Autodesk Inventor part; units mm, degrees
ref_plane "YZ Plane" through (0, 0, 0) normal (1, 0, 0) x (0, 1, 0)
ref_plane "XZ Plane" through (0, 0, 0) normal (0, 1, 0) x (-1, 0, 0)
ref_plane "XY Plane" through (0, 0, 0) normal (0, 0, 1) x (1, 0, 0)
sketch "草图1" plane through (0, 0, 0) normal (0, 0, 1) x (1, 0, 0)
  circle A0 centre (0, 0) radius 15
  circle A1 centre (0, 150) radius 5
  line L0 (0, 150) -> (0, 0)
  line L1 (-14.96663, 1) -> (-4.988877, 150.333333)
  line L2 (4.988877, 150.333333) -> (14.96663, 1)
  dimension "d0" = 30
  dimension "d1" = 10
  dimension "d2" = 150
extrude "拉伸1" add sketch "草图1" along normal blind 15
sketch "草图2" plane through (0, 0, 15) normal (0, 0, 1) x (1, 0, 0)
  circle A0 centre (0, 0) radius 7.5
  dimension "d5" = 15
extrude "拉伸2" cut sketch "草图2" against normal through all
sketch "草图3" plane through (0, 0, 15) normal (0, 0, 1) x (1, 0, 0)
  circle A0 centre (0, 150) radius 5
  arc A1 (4.988877, 150.333333) -> (-4.988877, 150.333333) centre (0, 150) ccw
  point P0 (0, 0)
  dimension "d8" = 10
extrude "拉伸3" add sketch "草图3" along normal blind 42.5
thread "螺纹1"
chamfer "倒角1" distance 0.25 angle 45 1 edges at (-5, 150, 57.5)
chamfer "倒角2" distance 1 angle 45 7 edges at (9.9778, 75.6667, 15) (0, -15, 15) (-9.9778, 75.6667, 15) (9.9778, 75.6667, 0) (0, 155, 0) (-9.9778, 75.6667, 0) (0, -15, 0)
chamfer "倒角3" distance 0.25 angle 45 1 edges at (-5, 150, 57.25)
equation "\"d6\" = d5"
properties part number "刀轴带动盘连杆"
Source: CAD feature listing. Evaluate the final solid. Frame: model axes, mm. A direction names the side the tool comes from. Coordinates: 2 decimals unless noted, no trailing zeros. Write each loop counter-clockwise with the first axis right and the second up, starting at its lowest first coordinate (ties: lowest second). Pieces come first, ordered by that corner, then holes. Notation, with made-up numbers: (-35, 85) -> (-6, 85) arc R30 cw to (-6, 115) -> close; hole circle Ø4 at (-27, 52). An arc over 180 degrees is marked (long way). Return JSON: item names as keys, results as strings. Group by question number.
1) Section query B-B, the plane y = 31. Return loops of the section in (x, z), plus the area to 3 significant figures.
2) Contact query for flat-ended pins moving along their axis: P1, Ø1.5, axis at y = 29.5, z = 10.5, coming from the -X side; P2, Ø1, axis at x = -6.5, y = 131, coming from the -Z side; P3, Ø8, axis at x = -11.5, y = 3, coming from the +Z side. Output: stop coordinate, or through.
3) Section query C-C, the plane z = 30. Return loops of the section in (x, y), plus the area to 3 significant figures.
4) Section query A-A, the plane z = 7.5. Return loops of the section in (x, y), plus the area to 3 significant figures.
5) Set-up query: faces 1 (the face through (0, 150, 57.5)), 2 (the face through (2.26, 154.46, 28.61)). Return all of +Z, -Z, +X, -X, +Y, -Y with unobstructed straight access to the full face (end or side cutting, diameter ignored); none if empty.
6) Mould query, pull axis X, two halves, no side actions, for faces 3 (the face through (-7.493, 0.33, 7.605)), 4 (the face through (0.325, -14.17, 14.826)), 5 (the face through (9.91, 76.71, 7.41)), 6 (the face through (0, 50, 15)). Classes: +X half, -X half, draft (parallel to the pull), parting line (faces both ways), or undercut.
7) Section query D-D, the plane y = 54.5. Return loops of the section in (x, z).
8) Ray query, line 1 along Y through (x, z) = (0, 3); line 2 along Z through (x, y) = (-5.25, 6); line 3 along Y through (x, z) = (-0.25, 47). Return the intervals inside material, ascending.
From the geometry:
{
 "1": {"outline": "(-12.96, 1) -> (-11.96, 0) -> (11.96, 0) -> (12.96, 1) -> (12.96, 14) -> (11.96, 15) -> (-11.96, 15) -> (-12.96, 14) -> close", "area": "387 mm²"},
 "2": {"P1": "x = -13.11", "P2": "z = 0.72", "P3": "z = 15"},
 "3": {"outline": "circle Ø10 at (0, 150)", "area": "78.5 mm²"},
 "4": {"outline": "(-14.97, 1) arc R15 ccw (long way) to (14.97, 1) -> (4.99, 150.33) arc R5 ccw to (-4.99, 150.33) -> close; hole circle Ø15 at (0, 0)", "area": "3,220 mm²"},
 "5": {"face 1": "+Z, +X, -X, +Y, -Y", "face 2": "+Z"},
 "6": {"face 3": "undercut", "face 4": "parting line", "face 5": "+X half", "face 6": "draft"},
 "7": {"outline": "(-11.39, 1) -> (-10.39, 0) -> (10.39, 0) -> (11.39, 1) -> (11.39, 14) -> (10.39, 15) -> (-10.39, 15) -> (-11.39, 14) -> close"},
 "8": {"line 1": "-15 to -7.5, 7.5 to 155", "line 2": "0 to 15", "line 3": "145.01 to 154.99"}
}
